Design review of the part built by this model. Coordinates are the model's own, in mm. Face numbers are marked on the shaded views. Coordinates: 2 decimals unless noted, no trailing zeros. One line per item, written item: value.
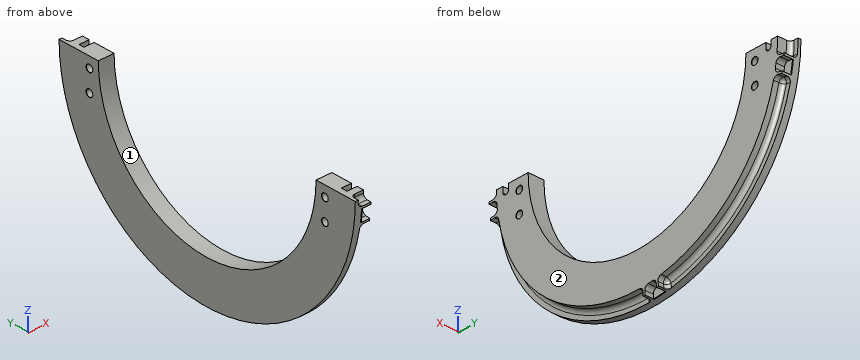
```python
from build123d import *

# Parameters (mm, degrees)
SKETCH1_W                         = 19.05
SKETCH1_H                         = 50.8
REVOLVE_THIN1_ANGLE               = 180
SKETCH81_W                        = 0.5
SKETCH81_H                        = 430
EXTRUDE1_DEPTH                    = 20.05
F_5_16_CLEARANCE_HOLE1_AT_2_COUNT = 2
F_5_16_CLEARANCE_HOLE1_AT_2_PITCH = 25.4
F_5_16_CLEARANCE_HOLE1_AT_3_COUNT = 2
F_5_16_CLEARANCE_HOLE1_AT_3_PITCH = 304.8
F_5_16_CLEARANCE_HOLE1_AT_4_COUNT = 2
F_5_16_CLEARANCE_HOLE1_AT_4_PITCH = 305.856502301
CUT_EXTRUDE1_DEPTH                = 11.311296
CUT_EXTRUDE2_DEPTH                = 4.175
BOSS_EXTRUDE1_DEPTH               = 1.064737
FILLET1_R                         = 4.7625
FILLET2_R                         = 4.7625
SKETCH90_W                        = 10
SKETCH90_H                        = 6.35254
CUT_EXTRUDE3_DEPTH                = 12.24534
SKETCH91_W                        = 10
SKETCH91_H                        = 7.35254
CUT_EXTRUDE4_DEPTH                = 12.24534
FILLET3_R                         = 3.175


with BuildPart() as part:
    # Sketch1 → Revolve-Thin1 (revolve)
    with BuildSketch(Plane.XY):
        with Locations((9.525, 166.3625)):
            Rectangle(SKETCH1_W, SKETCH1_H)
    revolve(axis=Axis((0, 0, 0), (-1, 0, 0)), revolution_arc=REVOLVE_THIN1_ANGLE)

    # Sketch81 → Extrude1 (cut, through all)
    with BuildSketch(Plane(origin=(0, 0, 0), x_dir=(0, 0, -1), z_dir=(1, 0, 0))):
        with Locations((0.25, 0)):
            Rectangle(SKETCH81_W, SKETCH81_H)
    extrude(amount=EXTRUDE1_DEPTH, mode=Mode.SUBTRACT)

    # Sketch83 → 5_16 Clearance Hole1 (revolve, cut)
    with BuildSketch(Plane(origin=(19.05, 152.4, -38.6), x_dir=(0, 0, -1), z_dir=(0, 1, 0))):
        Polygon((0, 0), (0, 19.05), (4.318, 19.05), (4.1021, 18.8341), (4.1021, 0.2159), (4.318, 0), align=None)
    f_5_16_clearance_hole1 = revolve(axis=Axis((25.4, 152.4, -38.6), (-1, 0, 0)), mode=Mode.SUBTRACT)

    # 5_16 Clearance Hole1 at 2: 5_16 Clearance Hole1 ×2
    with Locations(*[(0, 0, i * F_5_16_CLEARANCE_HOLE1_AT_2_PITCH) for i in range(1, F_5_16_CLEARANCE_HOLE1_AT_2_COUNT)]):
        add(f_5_16_clearance_hole1, mode=Mode.SUBTRACT)

    # 5_16 Clearance Hole1 at 3: 5_16 Clearance Hole1 ×2
    with Locations(*[(0, -i * F_5_16_CLEARANCE_HOLE1_AT_3_PITCH, 0) for i in range(1, F_5_16_CLEARANCE_HOLE1_AT_3_COUNT)]):
        add(f_5_16_clearance_hole1, mode=Mode.SUBTRACT)

    # 5_16 Clearance Hole1 at 4: 5_16 Clearance Hole1 ×2
    with Locations(*[Vector(0, -0.996545758, 0.08304548) * (i * F_5_16_CLEARANCE_HOLE1_AT_4_PITCH) for i in range(1, F_5_16_CLEARANCE_HOLE1_AT_4_COUNT)]):
        add(f_5_16_clearance_hole1, mode=Mode.SUBTRACT)

    # Sketch87 → Cut-Extrude1 (cut)
    with BuildSketch(Plane(origin=(19.05, 0, 0), x_dir=(0, 0, -1), z_dir=(1, 0, 0))):
        with BuildLine():
            Line((0.5, -181.961813044), (0.5, -191.761848151))
            ThreePointArc((0.5, -191.761848151), (4.660403781, -191.705860742), (8.818613515, -191.559621168))
            Line((8.818613515, -191.559621168), (8.367939309, -181.769989267))
            ThreePointArc((8.367939309, -181.769989267), (4.435006876, -181.908444335), (0.5, -181.961813044))
        make_face()
        with BuildLine():
            Line((0.5, 181.961813044), (0.5, 191.761848151))
            ThreePointArc((0.5, 191.761848151), (10.930348477, 191.450734886), (21.328330845, 190.572712395))
            Line((21.328330845, 190.572712395), (20.238349007, 180.833516351))
            ThreePointArc((20.238349007, 180.833516351), (10.384509774, 181.665938918), (0.5, 181.961813044))
        make_face()
        with BuildLine():
            Line((10.691988388, -181.648101533), (11.267829489, -191.431168896))
            ThreePointArc((11.267829489, -191.431168896), (18.796011872, -190.839111148), (26.295047079, -189.951117147))
            Line((26.295047079, -189.951117147), (24.951241792, -180.243687654))
            ThreePointArc((24.951241792, -180.243687654), (17.835443897, -181.086300827), (10.691988388, -181.648101533))
        make_face()
        with BuildLine():
            Line((27.254414037, -179.909833866), (28.72226185, -189.599282911))
            ThreePointArc((28.72226185, -189.599282911), (147.968659172, -121.975949716), (191.596275996, 7.982695695))
            Line((191.596275996, 7.982695695), (181.804770855, 7.574740971))
            ThreePointArc((181.804770855, 7.574740971), (140.406738255, -115.742383157), (27.254414037, -179.909833866))
        make_face()
        with BuildLine():
            Line((180.027040692, 26.469152346), (189.722802175, 27.894708123))
            ThreePointArc((189.722802175, 27.894708123), (140.246214207, 130.781710521), (41.061151684, 187.314810489))
            Line((41.061151684, 187.314810489), (38.962726359, 177.742109138))
            ThreePointArc((38.962726359, 177.742109138), (133.078947931, 124.098126593), (180.027040692, 26.469152346))
        make_face()
        with BuildLine():
            Line((22.54945028, 180.559889506), (23.763901679, 190.284348761))
            ThreePointArc((23.763901679, 190.284348761), (31.237243217, 189.201191969), (38.662144827, 187.824638862))
            Line((38.662144827, 187.824638862), (36.686320465, 178.225882792))
            ThreePointArc((36.686320465, 178.225882792), (29.640867578, 179.532087314), (22.54945028, 180.559889506))
        make_face()
        with BuildLine():
            Line((181.693024826, 9.89929976), (191.478511634, 10.43244883))
            ThreePointArc((191.478511634, 10.43244883), (190.919307311, 17.963142882), (190.064042372, 25.465981296))
            Line((190.064042372, 25.465981296), (180.350841849, 24.164545318))
            ThreePointArc((180.350841849, 24.164545318), (181.162398574, 17.045138579), (181.693024826, 9.89929976))
        make_face()
    extrude(amount=-CUT_EXTRUDE1_DEPTH, mode=Mode.SUBTRACT)

    # Sketch88 → Cut-Extrude2 (cut)
    with BuildSketch(Plane(origin=(7.738704, 0, 0), x_dir=(0, 0, -1), z_dir=(1, 0, 0))):
        with BuildLine():
            Line((8.818613515, -191.559621168), (8.367939309, -181.769989267))
            ThreePointArc((8.367939309, -181.769989267), (4.435006876, -181.908444335), (0.5, -181.961813044))
            Line((0.5, -181.961813044), (0.5, -191.761848151))
            ThreePointArc((0.5, -191.761848151), (4.660403781, -191.705860742), (8.818613515, -191.559621168))
        make_face()
        with BuildLine():
            Line((0.5, 191.761848151), (0.5, 181.961813044))
            ThreePointArc((0.5, 181.961813044), (10.384509774, 181.665938918), (20.238349007, 180.833516351))
            Line((20.238349007, 180.833516351), (21.328330845, 190.572712395))
            ThreePointArc((21.328330845, 190.572712395), (10.930348477, 191.450734886), (0.5, 191.761848151))
        make_face()
    extrude(amount=-CUT_EXTRUDE2_DEPTH, mode=Mode.SUBTRACT)

    # Sketch89 → Boss-Extrude1 (add)
    with BuildSketch(Plane(origin=(7.738704, 0, 0), x_dir=(0, 0, -1), z_dir=(1, 0, 0))):
        with BuildLine():
            Line((23.763901679, 190.284348761), (22.54945028, 180.559889506))
            ThreePointArc((22.54945028, 180.559889506), (29.640867578, 179.532087314), (36.686320465, 178.225882792))
            Line((36.686320465, 178.225882792), (38.662144827, 187.824638862))
            ThreePointArc((38.662144827, 187.824638862), (31.237243217, 189.201191969), (23.763901679, 190.284348761))
        make_face()
        with BuildLine():
            Line((190.064042372, 25.465981296), (180.350841849, 24.164545318))
            ThreePointArc((180.350841849, 24.164545318), (181.162398574, 17.045138579), (181.693024826, 9.89929976))
            Line((181.693024826, 9.89929976), (191.478511634, 10.43244883))
            ThreePointArc((191.478511634, 10.43244883), (190.919307311, 17.963142882), (190.064042372, 25.465981296))
        make_face()
        with BuildLine():
            Line((26.295047079, -189.951117147), (24.951241792, -180.243687654))
            ThreePointArc((24.951241792, -180.243687654), (17.835443897, -181.086300827), (10.691988388, -181.648101533))
            Line((10.691988388, -181.648101533), (11.267829489, -191.431168896))
            ThreePointArc((11.267829489, -191.431168896), (18.796011872, -190.839111148), (26.295047079, -189.951117147))
        make_face()
    extrude(amount=BOSS_EXTRUDE1_DEPTH)

    # Fillet1
    fillet1_edges = [part.edges().sort_by_distance(p)[0] for p in [
        (11.306852, -181.769989267, -8.367939309),
        (11.306852, 180.833516351, -20.238349007),
        (13.394352, -179.909833866, -27.254414037),
        (13.394352, 7.574740971, -181.804770855),
        (13.394352, 26.469152346, -180.027040692),
        (13.394352, 177.742109138, -38.962726359),
        (13.9267205, 180.559889506, -22.54945028),
        (13.9267205, 178.225882792, -36.686320465),
        (13.9267205, 24.164545318, -180.350841849),
        (13.9267205, 9.89929976, -181.693024826),
        (13.9267205, -180.243687654, -24.951241792),
        (13.9267205, -181.648101533, -10.691988388),
    ]]
    fillet(fillet1_edges, radius=FILLET1_R)

    # Fillet2
    fillet2_edges = [part.edges().sort_by_distance(p)[0] for p in [
        (7.738704, 7.876580746, -189.049363299),
        (7.738704, 184.824811835, -40.51532078),
        (3.563704, -189.013195727, -8.701386609),
        (3.563704, 181.783605025, -8.066743481),
        (3.563704, 188.039406053, -21.044810738),
        (3.563704, 182.35275146, -19.047706642),
        (7.738704, 124.098126593, -133.078947931),
        (7.738704, 27.523900361, -187.200793793),
        (7.738704, 28.007358428, -181.193070969),
        (7.738704, 178.797999192, -40.578523608),
        (3.563704, -181.950212254, -2.114631617),
        (3.563704, -183.20809984, -7.080483471),
        (7.738704, -187.078916486, -28.340453315),
        (7.738704, -115.742383157, -140.406738255),
        (7.738704, 6.281022467, -183.237250171),
        (7.738704, -181.069141374, -28.797693227),
    ]]
    fillet(fillet2_edges, radius=FILLET2_R)

    # Sketch90 → Cut-Extrude3 (cut)
    with BuildSketch(Plane(origin=(19.05, 0, 0), x_dir=(0, 0, -1), z_dir=(1, 0, 0))):
        with Locations((5.5, 170)):
            Rectangle(SKETCH90_W, SKETCH90_H)
        with Locations((5.5, -170)):
            Rectangle(SKETCH90_W, SKETCH90_H)
    extrude(amount=-CUT_EXTRUDE3_DEPTH, mode=Mode.SUBTRACT)

    # Sketch91 → Cut-Extrude4 (cut)
    with BuildSketch(Plane(origin=(19.05, 0, 0), x_dir=(0, 0, -1), z_dir=(1, 0, 0))):
        with Locations((5.5, -170)):
            Rectangle(SKETCH91_W, SKETCH91_H)
    extrude(amount=-CUT_EXTRUDE4_DEPTH, mode=Mode.SUBTRACT)

    # Fillet3
    fillet3_edges = [part.edges().sort_by_distance(p)[0] for p in [
        (12.92733, 173.17627, -10.5),
        (12.92733, 166.82373, -10.5),
        (12.92733, -166.32373, -10.5),
        (12.92733, -173.67627, -10.5),
    ]]
    fillet(fillet3_edges, radius=FILLET3_R)


solid = part.part
```
(1) We need section A-A on y = -152.4. State how many separate pieces and enclosed holes the cut face has, then the cut area to 3 significant figures.
Reply:
separate pieces: 3
enclosed holes: 0
area: 1,710 mm2
(2) Mouldability with a two-part tool opening along Y and no side actions: class the marked faces 1 and 2 as released by +Y, released by -Y, zero draft, split by the parting line, or undercut.
Reply:
face 1: undercut
face 2: zero draft
(3) To check wall thickness, follow line 1 along Z through (x, y) = (7.5, 152.4); line 2 along Z through (x, y) = (11.75, 152.4); line 3 along Y through (x, z) = (14.5, -13.2). State the ranges of each line that lie inside material, in increasing order. Write a range as [from, to].
Reply:
line 1: z = [-116.39, -42.7], [-34.5, -17.3], [-9.1, -0.5]
line 2: z = [-99.53, -42.7], [-34.5, -17.3], [-9.1, -0.5]
line 3: y = [-182.02, -156.5], [-148.3, -140.34], [140.34, 148.3], [156.5, 181.48]
(4) Insertion check: pin 1 (10 mm diameter, centred on x = 3.5, z = -159.5, fed in from -Y); pin 2 (6 mm diameter, centred on x = 14, y = -71, fed in from +Z); pin 3 (7.5 mm diameter, centred on x = 15.5, z = -2.5, fed in from -Y); pin 4 (12 mm diameter, centred on y = -32.5, z = -130.5, fed in from -X). Each pin has a flat end and moves straight along its axis. Give the tip position at first contact, or say it passes through.
Reply:
pin 1: stops at y = -113.59
pin 2: stops at z = -119.98
pin 3: stops at y = -182.59
pin 4: passes through
